Here's how the part is built. I have some questions about the finished solid (model axes, mm). Face numbers are marked on the shaded views. A direction names the side the tool comes from. Give positions to 0.01 mm unless a question says otherwise; leave off trailing zeros. Write each loop counter-clockwise with the first axis right and the second up, starting at its lowest first coordinate (ties: lowest second). Pieces come first, ordered by that corner, then holes. Notation, with made-up numbers: (17.25, 18) - (57.25, 18) arc R33 cw to (57.25, 48) - close; hole circle Ø10 at (-35, -24.5). An arc over 180 degrees is marked (long way). Use a Markdown table: item, result.
```python
from build123d import *

# Parameters (mm, degrees)
SKETCH1_W           = 196.85
SKETCH1_H           = 120.65
SKETCH1_R           = 3.175
BOSS_EXTRUDE2_DEPTH = 5.08
SKETCH4_W           = 171.45
SKETCH4_H           = 88.9
SKETCH4_W_2         = 151.638
SKETCH4_H_2         = 66.04
BOSS_EXTRUDE3_DEPTH = 25.4
FILLET4_R           = 12.7
CUT_EXTRUDE1_REACH  = 141.032
SKETCH7_W           = 50.8
SKETCH7_H           = 12.7


with BuildPart() as part:
    # Sketch1 → Boss-Extrude2 (new body)
    with BuildSketch(Plane(origin=(0, 0, 0), x_dir=(1, 0, 0), z_dir=(0, 1, 0))):
        Rectangle(SKETCH1_W, SKETCH1_H)
        with Locations(Location((-88.9, -50.8, 0), (0, 0, 270))):
            Circle(SKETCH1_R, mode=Mode.SUBTRACT)
        with Locations(Location((88.9, -50.8, 0), (0, 0, 270))):
            Circle(SKETCH1_R, mode=Mode.SUBTRACT)
        with Locations(Location((-88.9, 50.8, 0), (0, 0, 270))):
            Circle(SKETCH1_R, mode=Mode.SUBTRACT)
        with Locations(Location((88.9, 50.8, 0), (0, 0, 270))):
            Circle(SKETCH1_R, mode=Mode.SUBTRACT)
    extrude(amount=BOSS_EXTRUDE2_DEPTH)

    # Sketch4 → Boss-Extrude3 (add)
    with BuildSketch(Plane(origin=(0, 5.08, 0), x_dir=(1, 0, 0), z_dir=(0, 1, 0))):
        Rectangle(SKETCH4_W, SKETCH4_H)
        Rectangle(SKETCH4_W_2, SKETCH4_H_2, mode=Mode.SUBTRACT)
    extrude(amount=BOSS_EXTRUDE3_DEPTH)

    # Fillet4
    fillet4_edges = [part.edges().sort_by_distance(p)[0] for p in [
        (-85.725, 17.78, 44.45),
    ]]
    fillet(fillet4_edges, radius=FILLET4_R)

    # Sketch7 → Cut-Extrude1 (cut, up to next)
    with BuildSketch(Plane(origin=(0, 0, 33.02), x_dir=(-1, 0, 0), z_dir=(0, 0, -1)), mode=Mode.PRIVATE) as cut_extrude1_sk1:
        with Locations((3.176986547, 24.13)):
            Rectangle(SKETCH7_W, SKETCH7_H)
    cut_extrude1_tool1 = extrude(cut_extrude1_sk1.sketch, amount=-CUT_EXTRUDE1_REACH, mode=Mode.PRIVATE) & part.part
    add(cut_extrude1_tool1.solids().sort_by_distance((-3.176987, 24.13, 33.02))[0], mode=Mode.SUBTRACT)


solid = part.part
```
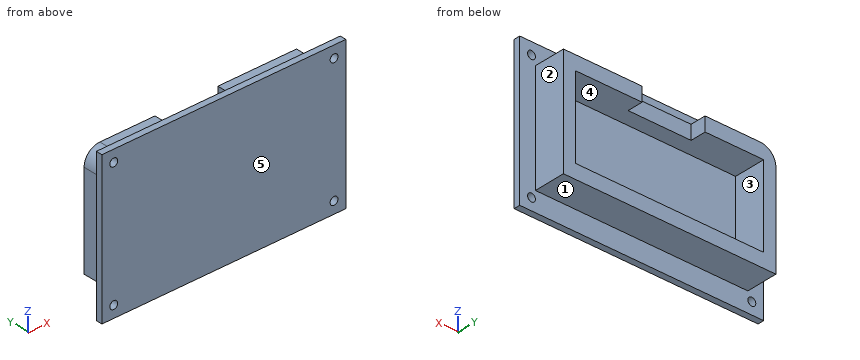
Item 1: For the marked faces 4 and 5, which set-ups out of +Z, -Z, +X, -X, +Y, -Y let a thin tool reach every point of the face, with its end or its side?
Values:
| item | result |
|---|---|
| face 4 | +Y |
| face 5 | +Z, -Z, +X, -X, -Y |
Item 2: Will these pins go through, and if not, where does the flat tip stop? pin 1 Ø1.5 at (y, z) = (22.5, -19) entering from +X (3 decimals); pin 2 Ø10 at (x, y) = (-56, 12.5) entering from +Z; pin 3 Ø7.5 at (y, z) = (14.5, 13.5) entering from -X (3 decimals).
Values:
| item | result |
|---|---|
| pin 1 | stops at x = 85.725 |
| pin 2 | stops at z = 44.45 |
| pin 3 | stops at x = -85.725 |
Item 3: If we section it at B-B, the plane z = -50.8: Write out the boundary of the cut face in (x, y) (3 decimals).
Values:
| item | result |
|---|---|
| outline | (-98.425, 0) - (-92.075, 0) - (-92.075, 5.08) - (-98.425, 5.08) - close; (-85.725, 0) - (85.725, 0) - (85.725, 5.08) - (-85.725, 5.08) - close; (92.075, 0) - (98.425, 0) - (98.425, 5.08) - (92.075, 5.08) - close |
Item 4: If we section it at A-A, the plane x = -88.9: Write out the boundary of the cut face in (y, z) (3 decimals).
Values:
| item | result |
|---|---|
| outline | (0, -60.325) - (5.08, -60.325) - (5.08, -53.975) - (0, -53.975) - close; (0, -47.625) - (5.08, -47.625) - (5.08, 47.625) - (0, 47.625) - close; (0, 53.975) - (5.08, 53.975) - (5.08, 60.325) - (0, 60.325) - close |
Item 5: If we section it at C-C, the plane y = 26.5: Write out the boundary of the cut face in (x, z) (3 decimals), plus the area to 3 significant figures.
Values:
| item | result |
|---|---|
| outline | (-85.725, -44.45) - (85.725, -44.45) - (85.725, 44.45) - (22.223, 44.45) - (22.223, 33.02) - (75.819, 33.02) - (75.819, -33.02) - (-75.819, -33.02) - (-75.819, 33.02) - (-28.577, 33.02) - (-28.577, 44.45) - (-73.025, 44.45) arc R12.7 ccw to (-85.725, 31.75) - close |
| area | 4,610 mm2 |
Item 6: I need wall thicknesses on line 1 along X through (y, z) = (2.5, -50.8) (3 decimals); line 2 along X through (y, z) = (25.5, -7) (3 decimals); line 3 along Z through (x, y) = (-1.5, 14). Which ranges of each line are inside material? Lowest first, please. Write a range as [from, to].
Values:
| item | result |
|---|---|
| line 1 | x = [-98.425, -92.075], [-85.725, 85.725], [92.075, 98.425] |
| line 2 | x = [-85.725, -75.819], [75.819, 85.725] |
| line 3 | z = [-44.45, -33.02], [33.02, 44.45] |
Item 7: If we section it at D-D, the plane z = 16: Write out the boundary of the cut face in (x, y) (3 decimals).
Values:
| item | result |
|---|---|
| outline | (-98.425, 0) - (98.425, 0) - (98.425, 5.08) - (85.725, 5.08) - (85.725, 30.48) - (75.819, 30.48) - (75.819, 5.08) - (-75.819, 5.08) - (-75.819, 30.48) - (-85.725, 30.48) - (-85.725, 5.08) - (-98.425, 5.08) - close |
Item 8: Thinking about a two-plate mould opening in Z: for the marked faces 1, 2 and 3, which applies, +Z half, -Z half, draft (parallel to the pull), parting line (faces both ways), or undercut?
Values:
| item | result |
|---|---|
| face 1 | -Z half |
| face 2 | draft |
| face 3 | undercut |
